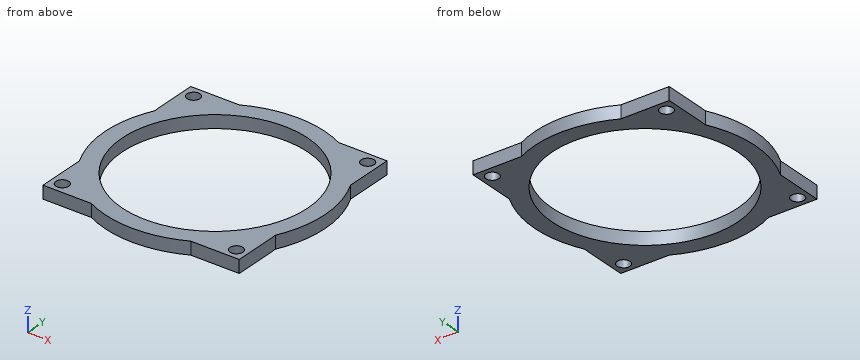
```python
from build123d import *

# Parameters (mm, degrees)
SKETCH1_R           = 1.5
SKETCH1_R_2         = 21.49615086
BOSS_EXTRUDE1_DEPTH = 3


with BuildPart() as part:
    # Sketch1 → Boss-Extrude1 (new body)
    # profile 1 of 2: a face of its own
    with BuildSketch(Plane.XY):
        with BuildLine():
            Line((22.75, -22.75), (22.75, -11.519006034))
            ThreePointArc((22.75, -11.519006034), (25.5, 0), (22.75, 11.519006034))
            Line((22.75, 11.519006034), (22.75, 22.75))
            Line((22.75, 22.75), (11.519006034, 22.75))
            ThreePointArc((11.519006034, 22.75), (0, 25.5), (-11.519006034, 22.75))
            Line((-11.519006034, 22.75), (-22.75, 22.75))
            Line((-22.75, 22.75), (-22.75, 11.519006034))
            ThreePointArc((-22.75, 11.519006034), (-18.03122292, -18.03122292), (11.519006034, -22.75))
            Line((11.519006034, -22.75), (22.75, -22.75))
        make_face()
        with Locations((20.207389371, 20.188817575)):
            Circle(SKETCH1_R, mode=Mode.SUBTRACT)
        with Locations((-20.188817575, 20.207389371)):
            Circle(SKETCH1_R, mode=Mode.SUBTRACT)
        with Locations((20.188817575, -20.207389371)):
            Circle(SKETCH1_R, mode=Mode.SUBTRACT)
        Circle(SKETCH1_R_2, mode=Mode.SUBTRACT)
    # profile 2 of 2: a face of its own
    with BuildSketch(Plane.XY):
        with BuildLine():
            Line((-22.75, -22.75), (-11.519006034, -22.75))
            ThreePointArc((-11.519006034, -22.75), (-18.03122292, -18.03122292), (-22.75, -11.519006034))
            Line((-22.75, -11.519006034), (-22.75, -22.75))
        make_face()
        with Locations((-20.207389371, -20.188817575)):
            Circle(SKETCH1_R, mode=Mode.SUBTRACT)
    extrude(amount=BOSS_EXTRUDE1_DEPTH)


solid = part.part
```
Part model, mm, in its own coordinate system. Coordinates: 2 decimals unless noted, no trailing zeros. Order: outer loops, then holes, each group sorted by start corner. A loop starts at its lowest first (then second) coordinate and runs counter-clockwise, first axis right, second up. Notation, with made-up numbers: (-33.5, 71.25) -> (-29.5, 71.25) arc R21 cw to (-29.5, 89.25) -> close; hole circle Ø9 at (0, -27.75). An arc over 180 degrees is marked (long way). Put each result on its own line as item: value. Start each with the question number.
(1) Band-saw the part on A-A (y = 0). Give the cut face in (x, z), then the cut area to 3 significant figures.
(2) Band-saw the part on C-C (z = 1.15). Give the cut face in (x, y).
(3) Pin check, flat tips, straight feed: pin 1 Ø1 at (y, z) = (-6, 2.5) entering from -X; pin 2 Ø1.5 at (y, z) = (-16, 1.5) entering from +X; pin 3 Ø1.5 at (y, z) = (-13, 1.5) entering from -X. Stop position of each tip, or through.
(4) Probe line 1 along Y through (x, z) = (19, 1.3); line 2 along X through (y, z) = (19, 0.9); line 3 along Y through (x, z) = (6, 0.5). List the from-to ranges inside material, lowest first. Write a range as [from, to].
Determined:
1. outline: (-25.5, 0) -> (-21.5, 0) -> (-21.5, 3) -> (-25.5, 3) -> close; (21.5, 0) -> (25.5, 0) -> (25.5, 3) -> (21.5, 3) -> close
1. area: 24.0 mm²
2. outline: (-22.75, -22.75) -> (-11.52, -22.75) arc R25.5 ccw to (11.52, -22.75) -> (22.75, -22.75) -> (22.75, -11.52) arc R25.5 ccw to (22.75, 11.52) -> (22.75, 22.75) -> (11.52, 22.75) arc R25.5 ccw to (-11.52, 22.75) -> (-22.75, 22.75) -> (-22.75, 11.52) arc R25.5 ccw to (-22.75, -11.52) -> close; hole circle Ø3 at (-20.21, -20.19); hole circle Ø3 at (-20.19, 20.21); hole circle Ø42.99 at (0, 0); hole circle Ø3 at (20.19, -20.21); hole circle Ø3 at (20.21, 20.19)
3. pin 1: stops at x = -24.9
3. pin 2: stops at x = 22.75
3. pin 3: stops at x = -22.75
4. line 1: y = [-22.75, -21.12], [-19.29, -10.05], [10.05, 19.3], [21.08, 22.75]
4. line 2: x = [-22.75, -21.08], [-19.3, -10.05], [10.05, 19.29], [21.12, 22.75]
4. line 3: y = [-24.78, -20.64], [20.64, 24.78]
